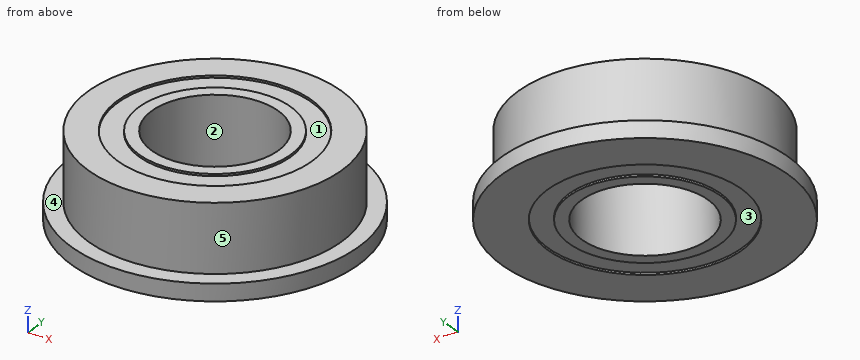
Autodesk Inventor part; units mm, degrees
ref_plane "YZ Plane" through (0, 0, 0) normal (1, 0, 0) x (0, 1, 0)
ref_plane "XZ Plane" through (0, 0, 0) normal (0, 1, 0) x (-1, 0, 0)
ref_plane "XY Plane" through (0, 0, 0) normal (0, 0, 1) x (1, 0, 0)
sketch "スケッチ1" plane through (0, 0, 0) normal (0, 0, 1) x (1, 0, 0)
  circle A0 centre (0, 0) radius 3
  circle A1 centre (0, 0) radius 6
  circle A2 centre (0, 0) radius 6.8
  dimension "d0" = 6
  dimension "d1" = 12
  dimension "d2" = 0.8
extrude "押し出し1" add sketch "スケッチ1" along normal blind 4 contours A1
extrude "押し出し2" add sketch "スケッチ1" along normal blind 0.8 contours A2
sketch "スケッチ2" plane through (0, 0, 0) normal (0, 0, -1) x (-1, 0, 0)
  circle A0 centre (0, 0) radius 3.6
  circle A1 centre (0, 0) radius 4.6
  dimension "d7" = 7.2
  dimension "d8" = 9.2
extrude "押し出し3" cut sketch "スケッチ2" against normal blind 0.1
sketch "スケッチ3" plane through (0, 0, 4) normal (0, 0, 1) x (1, 0, 0)
  circle A0 centre (0, 0) radius 3.6
  circle A1 centre (0, 0) radius 4.6
  dimension "d11" = 7.2
  dimension "d12" = 9.2
extrude "押し出し4" cut sketch "スケッチ3" against normal blind 0.1
properties part number "ベアリングFd6D12B4" material "鋼、炭素鋼"
Geometry check sheet. Reference: the model listing, model coordinates, mm. Face numbers are marked on the shaded views. A direction names the side the tool comes from. Round coordinates to 2 decimals unless told otherwise and drop trailing zeros. Order: outer loops, then holes, each group sorted by start corner. A loop starts at its lowest first (then second) coordinate and runs counter-clockwise, first axis right, second up. Notation, with made-up numbers: (39, -37.5) - (70, -37.5) arc R18 cw to (70, -22.5) - close; hole circle Ø5 at (-19.75, 64.5). An arc over 180 degrees is marked (long way). Use a Markdown table: item, result. Add a question column.
(1) Material ranges on line 1 along Y through (x, z) = (0, 3.95); line 2 along Y through (x, z) = (0, 2.55); line 3 along X through (y, z) = (-0.75, 0.85), recorded low to high. Write a range as [from, to].
(2) Depth check by flat-ended pin: pin 1 (5 mm diameter, centred on x = -5, y = 5, fed in from -Z); pin 2 (1.5 mm diameter, centred on x = 4.5, z = 2, fed in from -Y); pin 3 (5.5 mm diameter, centred on x = 0, y = 0, fed in from +Z); pin 4 (1.5 mm diameter, centred on x = 0, z = 2, fed in from +Y). Enter the tip coordinate at first touch or a pass-through.
(3) Sectioned sample at D-D, the plane z = 3.25. Enter the section's corners in (x, y).
(4) Sectioned sample at A-A, the plane x = 0. Enter the section's corners in (y, z).
(5) Release check for a two-part mould opening along Y. For the marked faces 3, 4 and 5 record: pulls with the +Y half, pulls with the -Y half, needs draft (parallel to the pull), parting line crosses it, or undercut.
(6) Sectioned sample at C-C, the plane x = -5.5. Enter the section's corners in (y, z).
(7) Tool access check on the marked faces 1 and 2. Record the directions out of +Z, -Z, +X, -X, +Y, -Y that give a thin tool (end or side, any length) a straight path to the whole face; none if there is none.
Answers below:
| question | item | result |
|---|---|---|
| 1 | line 1 | [-6, -4.6], [-3.6, -3], [3, 3.6], [4.6, 6] |
| 1 | line 2 | [-6, -3], [3, 6] |
| 1 | line 3 | [-5.95, -2.9], [2.9, 5.95] |
| 2 | pin 1 | z = 0 |
| 2 | pin 2 | y = -4.68 |
| 2 | pin 3 | through |
| 2 | pin 4 | y = 6 |
| 3 | outline | circle Ø12 at (0, 0); hole circle Ø6 at (0, 0) |
| 4 | outline | (-6.8, 0) - (-4.6, 0) - (-4.6, 0.1) - (-3.6, 0.1) - (-3.6, 0) - (-3, 0) - (-3, 4) - (-3.6, 4) - (-3.6, 3.9) - (-4.6, 3.9) - (-4.6, 4) - (-6, 4) - (-6, 0.8) - (-6.8, 0.8) - close; (3, 0) - (3.6, 0) - (3.6, 0.1) - (4.6, 0.1) - (4.6, 0) - (6.8, 0) - (6.8, 0.8) - (6, 0.8) - (6, 4) - (4.6, 4) - (4.6, 3.9) - (3.6, 3.9) - (3.6, 4) - (3, 4) - close |
| 5 | face 3 | undercut |
| 5 | face 4 | needs draft |
| 5 | face 5 | parting line crosses it |
| 6 | outline | (-4, 0) - (4, 0) - (4, 0.8) - (2.4, 0.8) - (2.4, 4) - (-2.4, 4) - (-2.4, 0.8) - (-4, 0.8) - close |
| 7 | face 1 | +Z |
| 7 | face 2 | +Z, -Z |
